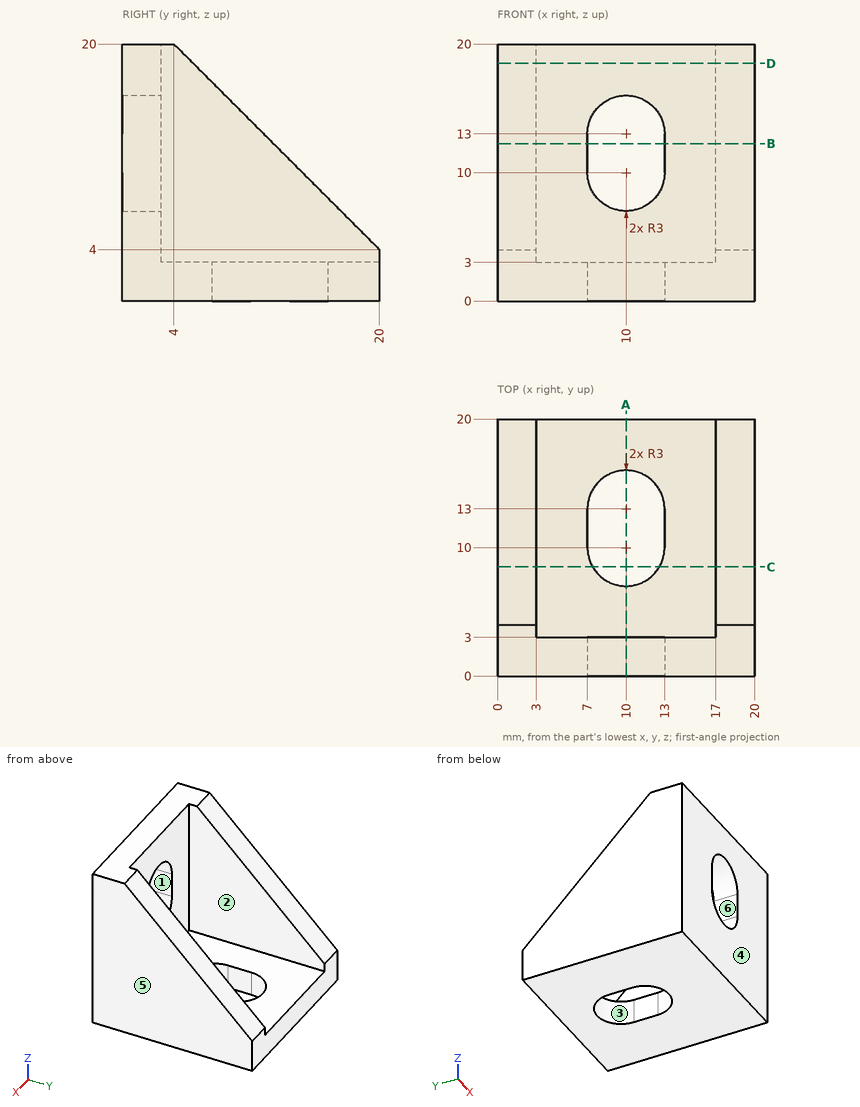
Can you work these out from the drawing? Everything is in mm from the part's minimum corner. A direction names the side the tool comes from. Round coordinates to 2 decimals unless told otherwise and drop trailing zeros. Write each loop counter-clockwise with the first axis right and the second up, starting at its lowest first coordinate (ties: lowest second). Pieces come first, ordered by that corner, then holes. Notation, with made-up numbers: (82.25, -14) - (119.25, -14) arc R5 ccw to (119.25, -8) - close; hole circle Ø8 at (68, -18.5). An arc over 180 degrees is marked (long way). Put each result on its own line as item: value. Start each with the question number.
(1) I want a section at B-B, the plane z = 12.25. Please give me the cut outline in (x, y), plus the area to 3 significant figures.
(2) For the marked faces 1, 2 and 3, which set-ups out of +Z, -Z, +X, -X, +Y, -Y let a thin tool reach every point of the face, with its end or its side?
(3) Will these pins go through, and if not, where does the flat tip stop? pin 1 (6 mm diameter, centred on x = 10.5, y = 17, fed in from -Z); pin 2 (6 mm diameter, centred on x = 7, z = 9.5, fed in from +Y); pin 3 (4 mm diameter, centred on x = 11.5, y = 17.5, fed in from +Z).
(4) I want a section at C-C, the plane y = 8.5. Please give me the cut outline in (x, z), plus the area to 3 significant figures.
(5) I want a section at D-D, the plane z = 18.5. Please give me the cut outline in (x, y), plus the area to 3 significant figures.
(6) I want a section at A-A, the plane x = 10. Please give me the cut outline in (y, z).
(7) Thinking about a two-plate mould opening in X: for the marked faces 4, 5 and 6, which applies, released by +X, released by -X, zero draft, split by the parting line, or undercut?
(8) I need wall thicknesses on probe 1 along X at (y, z) = (16.75, 5.75); probe 2 along Z at (x, y) = (6, 9.25); probe 3 along X at (y, z) = (2, 15). Which ranges of each line are inside material? Lowest first, please.
Here are the results:
1. outline: (0, 0) - (7, 0) - (7, 3) - (3, 3) - (3, 11.75) - (0, 11.75) - close; (13, 0) - (20, 0) - (20, 11.75) - (17, 11.75) - (17, 3) - (13, 3) - close
1. area: 94.5 mm^2
2. face 1: +Y, -Y
2. face 2: +Z, +Y
2. face 3: +Z, -Z
3. pin 1: stops at z = 0
3. pin 2: stops at y = 3
3. pin 3: stops at z = 3
4. outline: (0, 0) - (7.4, 0) - (7.4, 3) - (3, 3) - (3, 15.5) - (0, 15.5) - close; (12.6, 0) - (20, 0) - (20, 15.5) - (17, 15.5) - (17, 3) - (12.6, 3) - close
4. area: 119 mm^2
5. outline: (0, 0) - (20, 0) - (20, 5.5) - (17, 5.5) - (17, 3) - (3, 3) - (3, 5.5) - (0, 5.5) - close
5. area: 75.0 mm^2
6. outline: (0, 0) - (7, 0) - (7, 3) - (3, 3) - (3, 7) - (0, 7) - close; (0, 16) - (3, 16) - (3, 20) - (0, 20) - close; (16, 0) - (20, 0) - (20, 3) - (16, 3) - close
7. face 4: zero draft
7. face 5: released by +X
7. face 6: undercut
8. probe 1: x = 0 to 3, 17 to 20
8. probe 2: z = 0 to 3
8. probe 3: x = 0 to 7.76, 12.24 to 20
